The model under review builds one solid part; all positions refer to its coordinate system, in mm. A direction names the side the tool comes from. Give positions to 0.01 mm unless a question says otherwise; leave off trailing zeros. One line per item, written item: value. Start each with the question number.
Q1. To check wall thickness, follow line 1 along Z through (x, y) = (13, -216.5); line 2 along Y through (x, z) = (-36, 42.5); line 3 along X through (y, z) = (26.5, 82.5). State the ranges of each line that lie inside material, in increasing order. Write a range as from..to.
Q2. Mouldability with a two-part tool opening along X and no side actions: class faces 3 (the face through (-91.016, 159.192, 141.296)), 4 (the face through (-6, 0, 49)), 5 (the face through (-3, -380, 24)) as released by +X, released by -X, zero draft, split by the parting line, or undercut.
Q3. For pin 1 (8 mm diameter, centred on x = 26, y = -16.5, fed in from +Z); pin 2 (1 mm diameter, centred on y = 120.5, z = 38, fed in from +X); pin 3 (1.5 mm diameter, centred on x = 127, z = 19, fed in from +Y), all flat-tipped, find the tip position at first contact; note any pin that passes through.
Q4. For faces 1 (the face through (2, -254, 56.807)), 2 (the face through (29.243, 283.2, 150.476)), list the 3-axis set-ups (+Z, -Z, +X, -X, +Y, -Y) from which the entire face can be reached by the end or side of a thin tool; tool diameter is ignored.
```python
from build123d import *

# Parameters (mm, degrees)
F6_DEPTH  = 150
F11_DEPTH = 150


# Not quite as in the source:
# - a feature names something its author has since deleted; it is built from what else it names


with BuildPart() as f4:
    # F2 (on Front) → F4 section 0
    with BuildSketch(Plane.XZ):
        Polygon((145, 0), (150, 0), (150, 35), (140, 55), (110, 140), (90, 160), (0, 170), (-90, 160), (-110, 140), (-140, 55), (-150, 35), (-150, 0), (-145, 0), (-145, 33.8196601125), (-135.3886514877, 53.0423571371), (-105.6625113622, 137.2664208259), (-87.704664423, 155.2242677651), (0, 164.9692304788), (87.704664423, 155.2242677651), (105.6625113622, 137.2664208259), (135.3886514877, 53.0423571371), (145, 33.8196601125), align=None)
    # F3 (on offset) → F4 section 1
    with BuildSketch(Plane.XZ.offset(-360)):
        Polygon((105, 0), (110, 0), (110, 40), (100, 60), (90, 120), (70, 140), (0, 160), (-70, 140), (-90, 120), (-100, 60), (-110, 40), (-110, 0), (-105, 0), (-105, 38.8196601125), (-95.191631809, 58.4363964945), (-85.3314510321, 117.5974811561), (-67.3806149527, 135.5483172355), (0, 154.7999215077), (67.3806149527, 135.5483172355), (85.3314510321, 117.5974811561), (95.191631809, 58.4363964945), (105, 38.8196601125), align=None)
    loft()

    # F5 (on Right) → F6 (cut, symmetric)
    with BuildSketch(Plane.YZ):
        Polygon((190, 35.5667099357), (190, 0), (189.9669915438, -2.0382583607), (17.2620066122, -21.4886017568), (427.6157569008, -24.6490443013), (429.8257231712, 105.1867231727), (363.7629151344, 190.5601769686), (299.2246747017, 170.2331602573), align=None)
    extrude(amount=F6_DEPTH, both=True, mode=Mode.SUBTRACT)

    # F8 (on Front) → F9 section 0
    with BuildSketch(Plane.XZ):
        Polygon((-150, 0), (150, 0), (150, 35), (140, 55), (110, 140), (90, 160), (0, 170), (-90, 160), (-110, 140), (-140, 55), (-150, 35), align=None)
    # F7 (on offset) → F9 section 1
    with BuildSketch(Plane.XZ.offset(380)):
        Polygon((-75, 0), (75, 0), (75, 35), (65, 55), (110, 130), (90, 150), (0, 160), (-90, 150), (-110, 130), (-65, 55), (-75, 35), align=None)
    loft()

    # F10 (on Right) → F11 (cut, symmetric)
    with BuildSketch(Plane.YZ):
        with BuildLine():
            Line((-388.3555531502, 56.8068251014), (-124.2432887277, 56.8068251014))
            ThreePointArc((-124.2432887277, 56.8068251014), (-31.2629634759, 79.7343565579), (40.3992684554, 143.2602339406))
            Line((40.3992684554, 143.2602339406), (80.7762278766, 201.8068251014))
            Line((80.7762278766, 201.8068251014), (45.3817601157, 256.7874745919))
            Line((45.3817601157, 256.7874745919), (-388.3555531502, 199.957123117))
            Line((-388.3555531502, 199.957123117), (-388.3555531502, 56.8068251014))
        make_face()
    extrude(amount=F11_DEPTH, both=True, mode=Mode.SUBTRACT)


solid = f4.part
```
Solved:
1. line 1: 0..56.81
1. line 2: -380..0
1. line 3: -127.75..-122.46, 122.46..127.75
2. face 3: released by -X
2. face 4: undercut
2. face 5: zero draft
3. pin 1: z = 90.94
3. pin 2: x = 136.2
3. pin 3: y = 190
4. face 1: +Z, +X, -X, -Y
4. face 2: -Z, +X, -X, +Y
